For this review, take the finished solid that the model builds, in its own axes (mm). A direction names the side the tool comes from. Give positions to 0.01 mm unless a question says otherwise; leave off trailing zeros. Write each loop counter-clockwise with the first axis right and the second up, starting at its lowest first coordinate (ties: lowest second). Pieces come first, ordered by that corner, then holes. Notation, with made-up numbers: M 77,-36 L 104,-36 A26 cw 104,-1 Z; hole C 36,64 d10. An arc over 180 degrees is marked long. Write item = value, one per line.
```python
from build123d import *
from build123d import SkipClean  # not in build123d's __all__

# Parameters (mm, degrees)
F2_FACE_R    = 83.9113721036
F2_FACE_R_2  = 12.7043497663
F3_DEPTH     = 6.35
F2_FACE1_R   = 83.9113721036
F2_FACE1_R_2 = 12.7043497663
F4_DEPTH     = 6.35
F5_R         = 22.8643497663
F5_R_2       = 12.7043497663
F6_DEPTH     = 38.1
F8_D         = 5.1054
F8_DEPTH     = 84.2447919947


# Not quite as in the source:
# - after a boolean that leaves OpenCascade's solid faulty, fix() repairs it


with BuildPart() as f2:
    # F0 (on Top) → F2 (revolve)
    with BuildSketch(Plane.XY):
        Polygon((71.2107136504, 12.2464282371), (0, 12.2464282371), (0, -10.1297611803), (71.2107136504, -10.1297611803), (55.7892807321, -3.7797611803), (55.7892807321, 5.8964282371), align=None)
    revolve(axis=Axis((-12.7, 0, -0.3324198911), (0, -1, 0)))

    # F2_face (on face) → F3 (join)
    with BuildSketch(Plane(origin=(-12.7, 12.2464282371, -0.3324198911), x_dir=(-1, 0, 0), z_dir=(0, 1, 0))):
        Circle(F2_FACE_R)
        Circle(F2_FACE_R_2, mode=Mode.SUBTRACT)
    with SkipClean():  # cleaning this boolean's faces spoils the solid; the shape is the same uncleaned
        extrude(amount=F3_DEPTH)

    # F2_face1 (on face) → F4 (join)
    with BuildSketch(Plane(origin=(-12.7, -10.1297611803, -0.3324198911), x_dir=(1, 0, 0), z_dir=(0, -1, 0))):
        Circle(F2_FACE1_R)
        Circle(F2_FACE1_R_2, mode=Mode.SUBTRACT)
    extrude(amount=F4_DEPTH)

    add(f2.part.fix(), mode=Mode.REPLACE)

    # F5 (on face) → F6 (join)
    with BuildSketch(Plane(origin=(0, 18.5964282371, 0), x_dir=(-1, 0, 0), z_dir=(0, 1, 0))):
        with Locations((12.7, -0.3324198911)):
            Circle(F5_R)
        with Locations((12.7, -0.3324198911)):
            Circle(F5_R_2, mode=Mode.SUBTRACT)
    extrude(amount=F6_DEPTH)

    # F8 (through all, one way)
    with BuildSketch(Plane.XY):
        with Locations((-11.8156038225, 40.2014479041)):
            Circle(F8_D / 2)
    extrude(amount=-F8_DEPTH, mode=Mode.SUBTRACT)


solid = f2.part
```
1. The part is to be moulded in two halves that separate along X. For faces 1 (the face through (-12.37, 37.71, -17.81)), 2 (the face through (-79.29, -13.26, -51.39)), 3 (the face through (-23, 56.696, -10)), say which applies: +X half, -X half, draft (parallel to the pull), parting line (faces both ways), or undercut.
Responses:
face_1 = undercut
face_2 = parting line
face_3 = draft
2. Insertion check: P1, Ø10, axis at x = -15, y = 7, coming from the +Z side; P2, Ø8, axis at x = -48, y = 10.5, coming from the -Z side (3 decimals); P3, Ø8, axis at x = 15, z = -61, coming from the +Y side. Each pin has a flat end and moves straight along its axis. Give the tip position at first contact, or say it passes through.
Responses:
P1 = 82.95
P2 = -78.025
P3 = 18.6
3. Machinability: for faces 4 (the face through (-30, 18.596, -18)), 5 (the face through (-14, -16.48, -18)), 6 (the face through (-21.95, 1.13, 67.53)), which of the approach directions +Z, -Z, +X, -X, +Y, -Y give a long, thin tool a straight path to every point of the face, cutting with its end or side? Answer none if there is none.
Responses:
face_4 = +Y
face_5 = +Z, -Z, +X, -X, -Y
face_6 = none
4. For line 1 along Z through (x, y) = (-12, 35.5); line 2 along Y through (x, z) = (-70, 60.5); line 3 along Z through (x, y) = (-17, -8), list the stretches that pass through material, from the lowest coordinate up. Write a range as from..to.
Responses:
line_1 = -23.19..-13.02, 12.35..22.52
line_2 = -16.48..-9.99, 12.11..18.6
line_3 = -78.95..-12.29, 11.62..78.29
5. We need section A-A, the plane y = 31.5. Write out the cut boundary in (x, z).
Responses:
outline = C -12.7,-0.33 d45.73; hole C -12.7,-0.33 d25.41
